Verification items for the finished model (mm, model axes). A direction names the side the tool comes from. Give positions to 0.01 mm unless a question says otherwise; leave off trailing zeros. Write each loop counter-clockwise with the first axis right and the second up, starting at its lowest first coordinate (ties: lowest second). Pieces come first, ordered by that corner, then holes. Notation, with made-up numbers: (66, -2) -> (100, -2) arc R34 ccw to (100, 29) -> close; hole circle Ø1 at (22, 8). An arc over 180 degrees is marked (long way). Write item = value, one per line.
from build123d import *

# Parameters (mm, degrees)
SKETCH1_W                      = 60
SKETCH1_H                      = 118
BOSS_EXTRUDE1_DEPTH            = 4
SKETCH2_R                      = 2.5
BOSS_EXTRUDE2_DEPTH            = 10
SKETCH3_R                      = 1.075
SKETCH3_R_2                    = 1.5
CUT_EXTRUDE1_DEPTH             = 8
SKETCH4_W                      = 14
SKETCH4_H                      = 14
BOSS_EXTRUDE3_DEPTH            = 5
SKETCH5_W                      = 60
SKETCH5_H                      = 118
SKETCH5_W_2                    = 54
SKETCH5_H_2                    = 112
BOSS_EXTRUDE4_DEPTH            = 16
SKETCH10_W                     = 62
SKETCH10_H                     = 120
SKETCH10_W_2                   = 60
SKETCH10_H_2                   = 118
BOSS_EXTRUDE7_DEPTH            = 20
SKETCH6_R                      = 1.5
CUT_EXTRUDE2_DEPTH             = 10
CUT_EXTRUDE3_REACH             = 63
SKETCH7_W                      = 5
SKETCH7_H                      = 10
CUT_EXTRUDE3_DIRECTION_2_DEPTH = 10
SKETCH8_R                      = 3
BOSS_EXTRUDE5_DEPTH            = 4


with BuildPart() as part:
    # Sketch1 → Boss-Extrude1 (new body)
    with BuildSketch(Plane(origin=(0, 0, 0), x_dir=(1, 0, 0), z_dir=(0, 1, 0))):
        Rectangle(SKETCH1_W, SKETCH1_H)
    extrude(amount=BOSS_EXTRUDE1_DEPTH)

    # Sketch2 → Boss-Extrude2 (add)
    with BuildSketch(Plane(origin=(0, 4, 0), x_dir=(1, 0, 0), z_dir=(0, 1, 0))):
        with Locations((-21.18316549, 52.849664436)):
            Circle(SKETCH2_R)
        with Locations((6.566834506, 52.850079416)):
            Circle(SKETCH2_R)
        with Locations((-21.449381738, -52.75)):
            Circle(SKETCH2_R)
        with Locations((6.300617416, -52.75)):
            Circle(SKETCH2_R)
        with Locations((11.396968897, -36.250000429)):
            Circle(SKETCH2_R)
        with Locations((11.400617416, -51.75)):
            Circle(SKETCH2_R)
    extrude(amount=BOSS_EXTRUDE2_DEPTH)

    # Sketch3 → Cut-Extrude1 (cut)
    with BuildSketch(Plane(origin=(0, 14, 0), x_dir=(1, 0, 0), z_dir=(0, 1, 0))):
        with Locations((-21.18316549, 52.849664436)):
            Circle(SKETCH3_R)
        with Locations((6.566834506, 52.850079416)):
            Circle(SKETCH3_R)
        with Locations((11.396968897, -36.250000429)):
            Circle(SKETCH3_R_2)
        with Locations((11.400617416, -51.75)):
            Circle(SKETCH3_R_2)
        with Locations((6.300617416, -52.75)):
            Circle(SKETCH3_R)
        with Locations((-21.449381738, -52.75)):
            Circle(SKETCH3_R)
    extrude(amount=-CUT_EXTRUDE1_DEPTH, mode=Mode.SUBTRACT)

    # Sketch4 → Boss-Extrude3 (add)
    with BuildSketch(Plane(origin=(0, 4, 0), x_dir=(1, 0, 0), z_dir=(0, 1, 0))):
        with Locations((19, -20.184694787)):
            Rectangle(SKETCH4_W, SKETCH4_H)
    extrude(amount=BOSS_EXTRUDE3_DEPTH)

    # Sketch5 → Boss-Extrude4 (add)
    with BuildSketch(Plane(origin=(0, 4, 0), x_dir=(1, 0, 0), z_dir=(0, 1, 0))):
        Rectangle(SKETCH5_W, SKETCH5_H)
        Rectangle(SKETCH5_W_2, SKETCH5_H_2, mode=Mode.SUBTRACT)
    extrude(amount=BOSS_EXTRUDE4_DEPTH)

    # Sketch10 → Boss-Extrude7 (add)
    with BuildSketch(Plane(origin=(0, 0, 0), x_dir=(1, 0, 0), z_dir=(0, 1, 0))):
        Rectangle(SKETCH10_W, SKETCH10_H)
        Rectangle(SKETCH10_W_2, SKETCH10_H_2, mode=Mode.SUBTRACT)
    extrude(amount=BOSS_EXTRUDE7_DEPTH)

    # Sketch6 → Cut-Extrude2 (cut)
    with BuildSketch(Plane(origin=(0, 20, 0), x_dir=(1, 0, 0), z_dir=(0, 1, 0))):
        with Locations((-28.5, 57.5)):
            Circle(SKETCH6_R)
        with Locations((28.5, 57.5)):
            Circle(SKETCH6_R)
        with Locations((-28.5, -57.5)):
            Circle(SKETCH6_R)
        with Locations((28.5, -57.5)):
            Circle(SKETCH6_R)
    extrude(amount=-CUT_EXTRUDE2_DEPTH, mode=Mode.SUBTRACT)

    # Sketch7 → Cut-Extrude3 (cut, up to next)
    with BuildSketch(Plane(origin=(30, 0, 0), x_dir=(0, 0, -1), z_dir=(1, 0, 0)), mode=Mode.PRIVATE) as cut_extrude3_sk1:
        with Locations((0, 20)):
            Rectangle(SKETCH7_W, SKETCH7_H)
    cut_extrude3_tool1 = extrude(cut_extrude3_sk1.sketch, amount=-CUT_EXTRUDE3_REACH, mode=Mode.PRIVATE) & part.part
    add(cut_extrude3_tool1.solids().sort_by_distance((30, 20, 0))[0], mode=Mode.SUBTRACT)

    # Sketch7 → Cut-Extrude3 direction 2 (cut)
    with BuildSketch(Plane(origin=(30, 0, 0), x_dir=(0, 0, -1), z_dir=(1, 0, 0))):
        with Locations((0, 20)):
            Rectangle(SKETCH7_W, SKETCH7_H)
    extrude(amount=CUT_EXTRUDE3_DIRECTION_2_DEPTH, mode=Mode.SUBTRACT)

    # Sketch8 → Boss-Extrude5 (add)
    with BuildSketch(Plane(origin=(0, 0, 0), x_dir=(1, 0, 0), z_dir=(0, 1, 0))):
        with BuildLine():
            Line((10, 59), (-10, 59))
            ThreePointArc((-10, 59), (0, 69), (10, 59))
        make_face()
        with Locations((0, 64)):
            Circle(SKETCH8_R, mode=Mode.SUBTRACT)
        with BuildLine():
            Line((7.946608606, -59.003318261), (-12.053391394, -59.003318261))
            ThreePointArc((-12.053391394, -59.003318261), (-2.053391394, -69.003318261), (7.946608606, -59.003318261))
        make_face()
        with Locations((-2.053391394, -64.003318261)):
            Circle(SKETCH8_R, mode=Mode.SUBTRACT)
    extrude(amount=BOSS_EXTRUDE5_DEPTH)


solid = part.part
Item 1: Sectioned sample at B-B on x = -17. Record the cut outline in (y, z), then the cut area to 3 significant figures.
Response values:
outline = (0, -60) -> (20, -60) -> (20, -56) -> (4, -56) -> (4, 56) -> (20, 56) -> (20, 60) -> (0, 60) -> close
area = 608 mm^2
Item 2: Sectioned sample at A-A on z = 29. Record the cut outline in (x, y), then the cut area to 3 significant figures.
Response values:
outline = (-31, 0) -> (31, 0) -> (31, 20) -> (27, 20) -> (27, 4) -> (-27, 4) -> (-27, 20) -> (-31, 20) -> close
area = 376 mm^2
Item 3: Go/stop test with flat-tipped pins: P1, Ø1.5, axis at x = 11, z = 36.5, coming from the +Y side; P2, Ø2, axis at x = 1.5, y = 16.5, coming from the -Z side; P3, Ø10, axis at x = -18.5, z = -46, coming from the +Y side. Record where each tip stops, or that it passes through.
Response values:
P1 = 6
P2 = -60
P3 = 14
Item 4: Set-up check for faces 5 (the flat face through (29, 17, 2.5)), 6 (the cylindrical face through (-0.65, 1.97, -61.07)), 7 (the cylindrical face through (5.8, 8.9, 55.2)): record each of +Z, -Z, +X, -X, +Y, -Y from which the full face is reachable in a straight line by a thin tool's end or side.
Response values:
face_5 = +X, +Y
face_6 = +Y, -Y
face_7 = +Y
Item 5: Material ranges on line 1 (Z direction, x = 19, y = 5); line 2 (Z direction, x = 28.5, y = 18.25); line 3 (Z direction, x = -28.5, y = 16.75), recorded low to high.
Response values:
line_1 = -60 to -56, 13.18 to 27.18, 56 to 60
line_2 = -60 to -59, -56 to -2.5, 2.5 to 56, 59 to 60
line_3 = -60 to -59, -56 to 56, 59 to 60
Item 6: Sectioned sample at D-D on x = 28.5. Record the cut outline in (y, z), then the cut area to 4 significant figures.
Response values:
outline = (0, -60) -> (20, -60) -> (20, -59) -> (10, -59) -> (10, -56) -> (20, -56) -> (20, -2.5) -> (15, -2.5) -> (15, 2.5) -> (20, 2.5) -> (20, 56) -> (10, 56) -> (10, 59) -> (20, 59) -> (20, 60) -> (0, 60) -> close
area = 2,315 mm^2
Item 7: Mould release check, pull along Z, two halves, no side actions. Record for faces 1 (the flat face through (0, 10, 60)), 2 (the flat face through (0, 12, -56)), 3 (the flat face through (29, 15, 0)), 4 (the flat face through (31, 10, 1)): +Z half, -Z half, draft (parallel to the pull), parting line (faces both ways), or undercut.
Response values:
face_1 = +Z half
face_2 = undercut
face_3 = undercut
face_4 = draft
Item 8: Sectioned sample at C-C on z = -64. Record the cut outline in (x, y).
Response values:
outline = (-8.66, 0) -> (-3, 0) -> (-3, 4) -> (-8.66, 4) -> close; (3, 0) -> (8.66, 0) -> (8.66, 4) -> (3, 4) -> close
